CAD build for the part. Positions are in the model's coordinates, mm. Round coordinates to 2 decimals unless told otherwise and drop trailing zeros. Write each loop counter-clockwise with the first axis right and the second up, starting at its lowest first coordinate (ties: lowest second). Pieces come first, ordered by that corner, then holes. Notation, with made-up numbers: (15.5, 16.25) - (37.5, 16.25) arc R9 ccw to (37.5, 23.25) - close; hole circle Ø1 at (2, 54.5). An arc over 180 degrees is marked (long way). Put each result on its own line as item: value. Start each with the question number.
Item 1: Pin check, flat tips, straight feed: pin 1 Ø0.9 at (y, z) = (1, -14.5) entering from +X; pin 2 Ø4 at (x, z) = (2, -38.5) entering from -Y. Stop position of each tip, or through.
Item 2: Cut at A-A (x = 0). Give the cut face in (y, z).
Item 3: Cut at B-B (z = -21.5). Give the cut face in (x, y).
Item 4: Drill centre lines: line 1 (Z direction, x = 9.5, y = 0.2); line 2 (Z direction, x = -9.25, y = 2.6); line 3 (X direction, y = 1.85, z = -7.5). Where is each one in solid material? Low to high. Write a range as from..to.
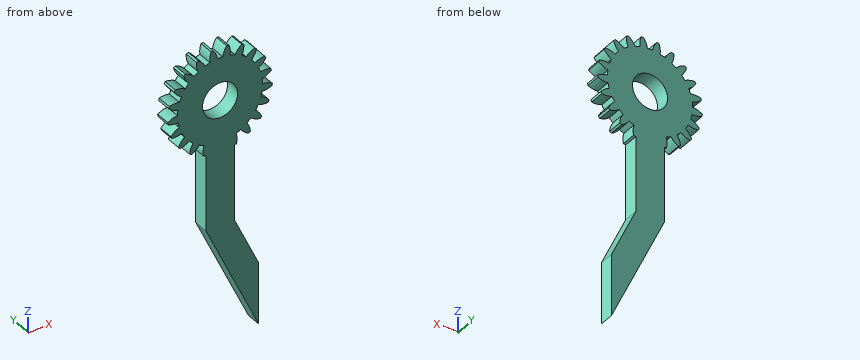
```python
from build123d import *

# Parameters (mm, degrees)
SKETCH1_R           = 3.5
BOSS_EXTRUDE1_DEPTH = 3
BOSS_EXTRUDE2_DEPTH = 3


with BuildPart() as part:
    # Sketch1 → Boss-Extrude1 (new body)
    with BuildSketch(Plane(origin=(0, 0, 0), x_dir=(1, 0, 0), z_dir=(0, 1, 0))):
        with BuildLine():
            Line((0.22, 10.45), (-0.22, 10.45))
            ThreePointArc((-0.22, 10.45), (-0.619608599, 9.494397866), (-0.75, 8.466847111))
            ThreePointArc((-0.75, 8.466847111), (-1.266859262, 8.405062023), (-1.778967393, 8.311755231))
            ThreePointArc((-1.778967393, 8.311755231), (-2.206441771, 9.255221249), (-2.869965555, 10.050581959))
            Line((-2.869965555, 10.050581959), (-3.29041759, 9.920889682))
            ThreePointArc((-3.29041759, 9.920889682), (-3.390604026, 8.889955567), (-3.212326601, 7.869622469))
            ThreePointArc((-3.212326601, 7.869622469), (-3.688011782, 7.658235377), (-4.149865725, 7.418127423))
            ThreePointArc((-4.149865725, 7.418127423), (-4.836440108, 8.193677608), (-5.704922076, 8.758125604))
            Line((-5.704922076, 8.758125604), (-6.068467137, 8.510264779))
            ThreePointArc((-6.068467137, 8.510264779), (-5.860329406, 7.495601704), (-5.389223887, 6.573147336))
            ThreePointArc((-5.389223887, 6.573147336), (-5.781468271, 6.230940911), (-6.152030277, 5.865366439))
            ThreePointArc((-6.152030277, 5.865366439), (-7.036699516, 6.404089754), (-8.032971235, 6.687471356))
            Line((-8.032971235, 6.687471356), (-8.307306748, 6.343465503))
            ThreePointArc((-8.307306748, 6.343465503), (-7.809338801, 5.435230735), (-7.08726498, 4.692619216))
            ThreePointArc((-7.08726498, 4.692619216), (-7.361215932, 4.25), (-7.607559941, 3.791441908))
            ThreePointArc((-7.607559941, 3.791441908), (-8.611717292, 4.045470421), (-9.647255648, 4.022605929))
            Line((-9.647255648, 4.022605929), (-9.808005699, 3.61302148))
            ThreePointArc((-9.808005699, 3.61302148), (-9.064454173, 2.891915663), (-8.155571478, 2.395131285))
            ThreePointArc((-8.155571478, 2.395131285), (-8.286887254, 1.891427939), (-8.387124519, 1.380631125))
            ThreePointArc((-8.387124519, 1.380631125), (-9.421546195, 1.327393289), (-10.40433906, 1.000314313))
            Line((-10.40433906, 1.000314313), (-10.437220301, 0.561544643))
            ThreePointArc((-10.437220301, 0.561544643), (-9.514153012, 0.091641193), (-8.499219659, -0.115174571))
            ThreePointArc((-8.499219659, -0.115174571), (-8.476232276, -0.635205795), (-8.421456277, -1.152854793))
            ThreePointArc((-8.421456277, -1.152854793), (-9.394229373, -1.508628563), (-10.236951288, -2.110859619))
            Line((-10.236951288, -2.110859619), (-10.139042077, -2.539827901))
            ThreePointArc((-10.139042077, -2.539827901), (-9.118477605, -2.716775998), (-8.087674876, -2.615246661))
            ThreePointArc((-8.087674876, -2.615246661), (-7.912426863, -3.105398707), (-7.707504688, -3.583904503))
            ThreePointArc((-7.707504688, -3.583904503), (-8.532194045, -4.210602146), (-9.15996547, -5.034474411))
            Line((-9.15996547, -5.034474411), (-8.93996547, -5.415525589))
            ThreePointArc((-8.93996547, -5.415525589), (-7.912585446, -5.28379572), (-6.957504688, -4.882942608))
            ThreePointArc((-6.957504688, -4.882942608), (-6.645567601, -5.299663316), (-6.308707484, -5.69650857))
            ThreePointArc((-6.308707484, -5.69650857), (-6.912035833, -6.53844525), (-7.269076522, -7.510754058))
            Line((-7.269076522, -7.510754058), (-6.946533698, -7.810030063))
            ThreePointArc((-6.946533698, -7.810030063), (-6.003625347, -7.381327005), (-5.209129676, -6.716767676))
            ThreePointArc((-5.209129676, -6.716767676), (-4.788220494, -7.023029582), (-4.349353934, -7.302952852))
            ThreePointArc((-4.349353934, -7.302952852), (-4.677712905, -8.285318801), (-4.732298225, -9.319670247))
            Line((-4.732298225, -9.319670247), (-4.335871923, -9.510579092))
            ThreePointArc((-4.335871923, -9.510579092), (-3.561216789, -8.822994992), (-2.997900632, -7.953778461))
            ThreePointArc((-2.997900632, -7.953778461), (-2.505418982, -8.122368849), (-2.0035412, -8.260497725))
            ThreePointArc((-2.0035412, -8.260497725), (-2.027754657, -9.296005416), (-1.775034463, -10.300492835))
            Line((-1.775034463, -10.300492835), (-1.3399489, -10.366071433))
            ThreePointArc((-1.3399489, -10.366071433), (-0.802378491, -9.480701156), (-0.520294961, -8.484061124))
            ThreePointArc((-0.520294961, -8.484061124), (0, -8.5), (0.520294961, -8.484061124))
            ThreePointArc((0.520294961, -8.484061124), (0.802378491, -9.480701156), (1.3399489, -10.366071433))
            Line((1.3399489, -10.366071433), (1.775034463, -10.300492835))
            ThreePointArc((1.775034463, -10.300492835), (2.027754657, -9.296005416), (2.0035412, -8.260497725))
            ThreePointArc((2.0035412, -8.260497725), (2.505418982, -8.122368849), (2.997900632, -7.953778461))
            ThreePointArc((2.997900632, -7.953778461), (3.561216789, -8.822994992), (4.335871923, -9.510579092))
            Line((4.335871923, -9.510579092), (4.732298225, -9.319670247))
            ThreePointArc((4.732298225, -9.319670247), (4.677712905, -8.285318801), (4.349353934, -7.302952852))
            ThreePointArc((4.349353934, -7.302952852), (4.788220494, -7.023029582), (5.209129676, -6.716767676))
            ThreePointArc((5.209129676, -6.716767676), (6.003625347, -7.381327005), (6.946533698, -7.810030063))
            Line((6.946533698, -7.810030063), (7.269076522, -7.510754058))
            ThreePointArc((7.269076522, -7.510754058), (6.912035833, -6.53844525), (6.308707484, -5.69650857))
            ThreePointArc((6.308707484, -5.69650857), (6.645567601, -5.299663316), (6.957504688, -4.882942608))
            ThreePointArc((6.957504688, -4.882942608), (7.912585446, -5.28379572), (8.93996547, -5.415525589))
            Line((8.93996547, -5.415525589), (9.15996547, -5.034474411))
            ThreePointArc((9.15996547, -5.034474411), (8.532194045, -4.210602146), (7.707504688, -3.583904503))
            ThreePointArc((7.707504688, -3.583904503), (7.912426863, -3.105398707), (8.087674876, -2.615246661))
            ThreePointArc((8.087674876, -2.615246661), (9.118477605, -2.716775998), (10.139042077, -2.539827901))
            Line((10.139042077, -2.539827901), (10.236951288, -2.110859619))
            ThreePointArc((10.236951288, -2.110859619), (9.394229373, -1.508628563), (8.421456277, -1.152854793))
            ThreePointArc((8.421456277, -1.152854793), (8.476232276, -0.635205795), (8.499219659, -0.115174571))
            ThreePointArc((8.499219659, -0.115174571), (9.514153012, 0.091641193), (10.437220301, 0.561544643))
            Line((10.437220301, 0.561544643), (10.40433906, 1.000314313))
            ThreePointArc((10.40433906, 1.000314313), (9.421546195, 1.327393289), (8.387124519, 1.380631125))
            ThreePointArc((8.387124519, 1.380631125), (8.286887254, 1.891427939), (8.155571478, 2.395131285))
            ThreePointArc((8.155571478, 2.395131285), (9.064454173, 2.891915663), (9.808005699, 3.61302148))
            Line((9.808005699, 3.61302148), (9.647255648, 4.022605929))
            ThreePointArc((9.647255648, 4.022605929), (8.611717292, 4.045470421), (7.607559941, 3.791441908))
            ThreePointArc((7.607559941, 3.791441908), (7.361215932, 4.25), (7.08726498, 4.692619216))
            ThreePointArc((7.08726498, 4.692619216), (7.809338801, 5.435230735), (8.307306748, 6.343465503))
            Line((8.307306748, 6.343465503), (8.032971235, 6.687471356))
            ThreePointArc((8.032971235, 6.687471356), (7.036699516, 6.404089754), (6.152030277, 5.865366439))
            ThreePointArc((6.152030277, 5.865366439), (5.781468271, 6.230940911), (5.389223887, 6.573147336))
            ThreePointArc((5.389223887, 6.573147336), (5.860329406, 7.495601704), (6.068467137, 8.510264779))
            Line((6.068467137, 8.510264779), (5.704922076, 8.758125604))
            ThreePointArc((5.704922076, 8.758125604), (4.836440108, 8.193677608), (4.149865725, 7.418127423))
            ThreePointArc((4.149865725, 7.418127423), (3.688011782, 7.658235377), (3.212326601, 7.869622469))
            ThreePointArc((3.212326601, 7.869622469), (3.390604026, 8.889955567), (3.29041759, 9.920889682))
            Line((3.29041759, 9.920889682), (2.869965555, 10.050581959))
            ThreePointArc((2.869965555, 10.050581959), (2.206441771, 9.255221249), (1.778967393, 8.311755231))
            ThreePointArc((1.778967393, 8.311755231), (1.266859262, 8.405062023), (0.75, 8.466847111))
            ThreePointArc((0.75, 8.466847111), (0.619608599, 9.494397866), (0.22, 10.45))
        make_face()
        with Locations(Location((0, 0, 0), (0, 0, 270))):
            Circle(SKETCH1_R, mode=Mode.SUBTRACT)
    extrude(amount=BOSS_EXTRUDE1_DEPTH)

    # Sketch4 → Boss-Extrude2 (add)
    with BuildSketch(Plane(origin=(0, 3, 0), x_dir=(1, 0, 0), z_dir=(0, 1, 0))):
        Polygon((-2.85, 4.257844413), (-2.85, 25), (7.715456544, 47.657694676), (7.715456544, 35.434005229), (2.85, 25), (2.85, 4.257844413), align=None)
    extrude(amount=-BOSS_EXTRUDE2_DEPTH)


solid = part.part
```
Output values:
1. pin 1: x = 2.85
1. pin 2: y = 0
2. outline: (0, -31.11) - (3, -31.11) - (3, -3.5) - (0, -3.5) - close; (0, 3.5) - (3, 3.5) - (3, 8.5) - (0, 8.5) - close
3. outline: (-2.85, 0) - (2.85, 0) - (2.85, 3) - (-2.85, 3) - close
4. line 1: -4.04..-3.27, -1.31..-0.09, 1.57..2.68
4. line 2: -4.06..-3.04, -1.36..-0.01, 1.44..2.71
4. line 3: -5.86..-4.21, -4..4, 4.21..5.86
